The model under review builds one solid part; all positions refer to its coordinate system, in mm. Round coordinates to 2 decimals unless told otherwise and drop trailing zeros. Loops run counter-clockwise (first coordinate to the right, second up) from the corner with the lowest first, then second, coordinate; pieces in that order, holes last. Notation, with made-up numbers: M 57.5,72.25 L 88.5,72.25 A33 cw 88.5,102.25 Z; hole C 8,27.5 d8. An arc over 180 degrees is marked long. Use a Markdown table: item, result. Add a question column.
```python
from build123d import *

# Parameters (mm, degrees)
MODEL_R             = 1.6
MODEL_R_2           = 2.5
BOSS_EXTRUDE1_DEPTH = 3


with BuildPart() as part:
    # Model → Boss-Extrude1 (new body)
    with BuildSketch(Plane.XY):
        with BuildLine():
            Line((146.020094854, 163.929669503), (146.020094854, 158.929672503))
            ThreePointArc((146.020094854, 158.929672503), (146.166539616, 158.576119306), (146.520091281, 158.429670848))
            Line((146.520091281, 158.429670848), (191.949370202, 158.429670848))
            ThreePointArc((191.949370202, 158.429670848), (193.533289392, 159.085751658), (194.189370202, 160.669670848))
            Line((194.189370202, 160.669670848), (194.189370202, 188.789666848))
            ThreePointArc((194.189370202, 188.789666848), (193.533289392, 190.373586038), (191.949370202, 191.029666848))
            Line((191.949370202, 191.029666848), (149.020161786, 191.029666848))
            Line((149.020161786, 191.029666848), (149.020161786, 186.495697517))
            ThreePointArc((149.020161786, 186.495697517), (149.087148935, 186.245697179), (149.270161786, 186.062684219))
            ThreePointArc((149.270161786, 186.062684219), (149.373716972, 185.276118333), (148.587150624, 185.379670014))
            ThreePointArc((148.587150624, 185.379670014), (148.404138038, 185.562681651), (148.154138786, 185.629668517))
            Line((148.154138786, 185.629668517), (146.520109786, 185.629668517))
            ThreePointArc((146.520109786, 185.629668517), (146.166556395, 185.483221908), (146.020109786, 185.129668517))
            Line((146.020109786, 185.129668517), (146.020109786, 180.129671517))
            ThreePointArc((146.020109786, 180.129671517), (146.166554627, 179.776114895), (146.520109786, 179.629666517))
            Line((146.520109786, 179.629666517), (148.154138786, 179.629666517))
            ThreePointArc((148.154138786, 179.629666517), (148.404140189, 179.696653822), (148.587154607, 179.879666726))
            ThreePointArc((148.587154607, 179.879666726), (149.373734927, 179.983242082), (149.270155207, 179.196662336))
            ThreePointArc((149.270155207, 179.196662336), (149.087143628, 179.013649891), (149.02015667, 178.76365081))
            Line((149.02015667, 178.76365081), (149.02015667, 173.629671744))
            Line((149.02015667, 173.629671744), (151.82015667, 173.629671744))
            Line((151.82015667, 173.629671744), (151.82015667, 175.054680432))
            Line((151.82015667, 175.054680432), (156.020152766, 175.054680432))
            Line((156.020152766, 175.054680432), (156.020152766, 173.629670513))
            Line((156.020152766, 173.629670513), (159.020147427, 173.629670513))
            Line((159.020147427, 173.629670513), (159.020147427, 170.429672075))
            Line((159.020147427, 170.429672075), (156.020147427, 170.429672075))
            Line((156.020147427, 170.429672075), (156.020147427, 169.154680763))
            Line((156.020147427, 169.154680763), (151.820147427, 169.154680763))
            Line((151.820147427, 169.154680763), (151.820147427, 170.429672075))
            Line((151.820147427, 170.429672075), (149.020147427, 170.429672075))
            Line((149.020147427, 170.429672075), (149.020147427, 165.295696252))
            ThreePointArc((149.020147427, 165.295696252), (149.08713456, 165.045696208), (149.270147141, 164.862683385))
            ThreePointArc((149.270147141, 164.862683385), (149.373701806, 164.07611743), (148.587135527, 164.179669631))
            ThreePointArc((148.587135527, 164.179669631), (148.404130845, 164.362680921), (148.154138455, 164.429670848))
            Line((148.154138455, 164.429670848), (146.520087311, 164.429670848))
            ThreePointArc((146.520087311, 164.429670848), (146.166538715, 164.283220702), (146.020094854, 163.929669503))
        make_face()
        with Locations((173.68542699, 177.029665772)):
            Circle(MODEL_R, mode=Mode.SUBTRACT)
        with Locations((183.68542699, 177.029665772)):
            Circle(MODEL_R_2, mode=Mode.SUBTRACT)
    extrude(amount=BOSS_EXTRUDE1_DEPTH)


solid = part.part
```
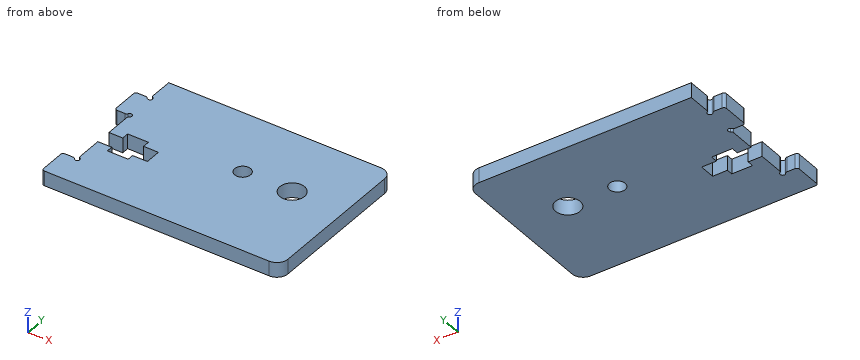
(1) Consider section A-A, the plane x = 182.5. Give the boundary of the cut face in (y, z), then the cut area to 3 significant figures.
(2) Consider section B-B, the plane z = 2.25. Give the number of separate pieces and of enclosed holes in the cut face, then the cut area to 3 significant figures.
(3) To check wall thickness, follow probe 1 along Y at (x, z) = (183.5, 0.3); probe 2 along Y at (x, z) = (155, 0.6); probe 3 along X at (y, z) = (166, 0.55). State the ranges of each line that lie inside material, in increasing order.
(4) Insertion check: pin 1 Ø0.8 at (x, z) = (147, 1.5) entering from +Y; pin 2 Ø1.5 at (y, z) = (176.5, 1.5) entering from -X; pin 3 Ø0.6 at (x, y) = (149.02, 164.43) entering from +Z. Each pin has a flat end and moves straight along its axis. Give the tip position at first contact, or say it passes through.
Found:
| question | item | result |
|---|---|---|
| 1 | outline | M 158.43,0 L 174.83,0 L 174.83,3 L 158.43,3 Z; M 179.23,0 L 191.03,0 L 191.03,3 L 179.23,3 Z |
| 1 | area | 84.6 mm^2 |
| 2 | separate pieces | 1 |
| 2 | enclosed holes | 2 |
| 2 | area | 1,430 mm^2 |
| 3 | probe 1 | y = 158.43 to 174.54, 179.52 to 191.03 |
| 3 | probe 2 | y = 158.43 to 169.15, 175.05 to 191.03 |
| 3 | probe 3 | x = 149.02 to 194.19 |
| 4 | pin 1 | stops at y = 185.63 |
| 4 | pin 2 | stops at x = 149.02 |
| 4 | pin 3 | passes through |
